from build123d import *

# Parameters (mm, degrees)
SKETCH1_W           = 51.89
SKETCH1_H           = 60
BOSS_EXTRUDE1_DEPTH = 3.175
CUT_EXTRUDE1_DEPTH  = 10


with BuildPart() as part:
    # Sketch1 → Boss-Extrude1 (new body)
    with BuildSketch(Plane(origin=(0, 0, 0), x_dir=(1, 0, 0), z_dir=(0, 1, 0))):
        Rectangle(SKETCH1_W, SKETCH1_H)
    extrude(amount=BOSS_EXTRUDE1_DEPTH)

    # Sketch2 → Cut-Extrude1 (cut)
    with BuildSketch(Plane(origin=(0, 3.175, 0), x_dir=(1, 0, 0), z_dir=(0, 1, 0))):
        Polygon((-3.5, 30), (3.5, 30), (3.5, 26.825), (1.47, 26.825), (1.47, 24.745), (3.25, 24.745), (3.25, 22.145), (1.47, 22.145), (1.47, 20.075), (-1.47, 20.075), (-1.47, 22.145), (-3.25, 22.145), (-3.25, 24.745), (-1.47, 24.745), (-1.47, 26.825), (-3.5, 26.825), align=None)
        Polygon((1.47, -26.825), (1.47, -24.745), (3.25, -24.745), (3.25, -22.145), (1.47, -22.145), (1.47, -20.075), (-1.47, -20.075), (-1.47, -22.145), (-3.25, -22.145), (-3.25, -24.745), (-1.47, -24.745), (-1.47, -26.825), (-3.5, -26.825), (-3.5, -30), (3.5, -30), (3.5, -26.825), align=None)
    extrude(amount=-CUT_EXTRUDE1_DEPTH, mode=Mode.SUBTRACT)


solid = part.part
Verification items for the finished model (mm, model axes). A direction names the side the tool comes from. Coordinates: 2 decimals unless noted, no trailing zeros. Write each loop counter-clockwise with the first axis right and the second up, starting at its lowest first coordinate (ties: lowest second). Pieces come first, ordered by that corner, then holes. Notation, with made-up numbers: M 20.25,-37 L 51.25,-37 A24 cw 51.25,-11 Z; hole C 33.25,41.25 d8. An arc over 180 degrees is marked long. One line per question, with ' | ' between items.
1) Release check for a two-part mould opening along Z. For faces 1 (the face through (15, 2, 30)), 2 (the face through (3.25, 2, -23)), 3 (the face through (0, 3.175, 0)) record: +Z half, -Z half, draft (parallel to the pull), parting line (faces both ways), or undercut.
Solutions:
face 1: +Z half | face 2: undercut | face 3: draft
2) Depth check by flat-ended pin: pin 1 Ø1.4 at (x, y) = (2.5, 1) entering from +Z (3 decimals); pin 2 Ø0.9 at (x, y) = (-2, 2) entering from -Z (3 decimals); pin 3 Ø0.9 at (x, y) = (0, 2) entering from -Z (3 decimals). Enter the tip coordinate at first touch or a pass-through.
Solutions:
pin 1: z = 26.825 | pin 2: z = -26.825 | pin 3: z = -20.075
3) Material ranges on L1, parallel to Z at x = 3, y = 1.8 (3 decimals); L2, parallel to X at y = 0.95, z = -26 (3 decimals); L3, parallel to X at y = 2.45, z = 22.5 (3 decimals), recorded low to high.
Solutions:
L1: -26.825 to -24.745, -22.145 to 22.145, 24.745 to 26.825 | L2: -25.945 to -1.47, 1.47 to 25.945 | L3: -25.945 to -3.25, 3.25 to 25.945
4) Access from +Z, -Z, +X, -X, +Y, -Y to the whole of each face (thin tool, end or side, straight path). Record for faces 4 (the face through (-2, 2, 26.825)), 5 (the face through (2, 2, -26.825)), 6 (the face through (-3.25, 2, 23)).
Solutions:
face 4: +Z, +Y, -Y | face 5: -Z, +Y, -Y | face 6: +Y, -Y
5) Sectioned sample at A-A on x = 0. Record the cut outline in (y, z) (3 decimals).
Solutions:
outline: M 0,-20.075 L 3.175,-20.075 L 3.175,20.075 L 0,20.075 Z
